For this review, take the finished solid that the model builds, in its own axes (mm). A direction names the side the tool comes from. Give positions to 0.01 mm unless a question says otherwise; leave off trailing zeros. Loops run counter-clockwise (first coordinate to the right, second up) from the corner with the lowest first, then second, coordinate; pieces in that order, holes last.
Autodesk Inventor part; units mm, degrees
ref_plane "YZ Plane" through (0, 0, 0) normal (1, 0, 0) x (0, 1, 0)
ref_plane "XZ Plane" through (0, 0, 0) normal (0, 1, 0) x (-1, 0, 0)
ref_plane "XY Plane" through (0, 0, 0) normal (0, 0, 1) x (1, 0, 0)
sketch "Esboço1" plane through (0, 0, 0) normal (1, 0, 0) x (0, 1, 0)
  line L0 (-24.5, 0) -> (24.5, 0) construction
  line L1 (0, -21) -> (0, 21) construction
  line L2 (-17.5, 15) -> (17.5, 15)
  line L3 (17.5, 15) -> (17.5, -15)
  line L4 (17.5, -15) -> (-17.5, -15)
  line L5 (-17.5, -15) -> (-17.5, 15)
  line L6 (-17.5, 15) -> (-1.5, 15)
  line L7 (-1.5, 15) -> (-1.5, 6)
  line L8 (-1.5, 6) -> (-17.5, 6)
  line L9 (-17.5, 6) -> (-17.5, 15)
  line L10 (-1.5, 15) -> (8.5, 15)
  line L11 (8.5, 15) -> (8.5, 11)
  line L12 (8.5, 11) -> (-1.5, 11)
  line L13 (-1.5, 11) -> (-1.5, 15)
  point P0 (0, 0)
  point P1 (8.5, 15)
  point P2 (-1.5, 11)
  point P3 (-17.5, 6)
  dimension "d0" = 35
  dimension "d1" = 30
  dimension "d3" = 16
  dimension "d5" = 10
  dimension "d16" = 4
  dimension "d17" = 9
extrude "Extrusão1" add sketch "Esboço1" along normal mid plane 10 contours L8 L7 L12 L11 L2 L3 L4 L5
sketch "Esboço2" plane through (5, 17.5, -15) normal (0, 0, -1) x (-1, 0, 0)
  point P0 (5, -17.5)
hole "Furo1" at (0, 0, -15) direction (0, 0, 1) diameter 3.242 depth 15 tip angle 118
chamfer "Chanfro1" distance 1 angle 45 4 edges at (0, -1.5, 11) (0, 8.5, 15) (0, 17.5, 15) (0, -17.5, 6)
properties part number "GRJ-05-102" material "Fenolite OR"
Q1. Mouldability with a two-part tool opening along Y and no side actions: class faces 4 (the flat face through (0, 8.5, 13)), 5 (the conical face through (-0.275, -0.061, 0.805)), 6 (the flat face through (0, 13, 15)), 7 (the flat face through (0, 17.5, 0)) as +Y half, -Y half, draft (parallel to the pull), parting line (faces both ways), or undercut.
Answers:
face 4: -Y half
face 5: undercut
face 6: draft
face 7: +Y half
Q2. Machinability: for faces 1 (the cylindrical face through (1.438, 0.748, -7.395)), 2 (the flat face through (-5, 0, -3)), 3 (the flat face through (0, 4, 11)), which of the approach directions +Z, -Z, +X, -X, +Y, -Y give a long, thin tool a straight path to every point of the face, cutting with its end or side? Answer none if there is none.
Answers:
face 1: -Z
face 2: +Z, -Z, -X, +Y, -Y
face 3: +Z, +X, -X, -Y
Q3. Consider section D-D on z = 7.25. Give the boundary of the cut face in (x, y), plus the area to 3 significant figures.
Answers:
outline: (-5, -1.5) - (5, -1.5) - (5, 17.5) - (-5, 17.5) - close
area: 190 mm2
Q4. For pin 1 Ø2.5 at (x, y) = (0, 0) entering from +Z; pin 2 Ø1.2 at (x, z) = (1.5, 8.5) entering from -Y; pin 3 Ø3.5 at (x, z) = (0, 12) entering from -Y, all flat-tipped, find the tip position at first contact; note any pin that passes through.
Answers:
pin 1: stops at z = 11
pin 2: stops at y = -1.5
pin 3: stops at y = -1.25
Q5. Consider section B-B on z = -7. Give the boundary of the cut face in (x, y), plus the area to 3 significant figures.
Answers:
outline: (-5, -17.5) - (5, -17.5) - (5, 17.5) - (-5, 17.5) - close; hole circle Ø3.24 at (0, 0)
area: 342 mm2
Q6. Consider section C-C on y = 5. Give the boundary of the cut face in (x, z), plus the area to 3 significant figures.
Answers:
outline: (-5, -15) - (5, -15) - (5, 11) - (-5, 11) - close
area: 260 mm2
Q7. For probe 1 along Y at (x, z) = (0, -6); probe 2 along X at (y, z) = (0, -4); probe 3 along Z at (x, y) = (4.25, -8), list the stretches that pass through material, from the lowest coordinate up.
Answers:
probe 1: y = -17.5 to -1.62, 1.62 to 17.5
probe 2: x = -5 to -1.62, 1.62 to 5
probe 3: z = -15 to 6
Q8. Consider section A-A on x = -4. Give the boundary of the cut face in (y, z), plus the area to 3 significant figures.
Answers:
outline: (-17.5, -15) - (17.5, -15) - (17.5, 14) - (16.5, 15) - (9.5, 15) - (8.5, 14) - (8.5, 11) - (-0.5, 11) - (-1.5, 10) - (-1.5, 6) - (-16.5, 6) - (-17.5, 5) - close
area: 864 mm2
